Verification items for this drawing (mm, ordinates from the low corner). A direction names the side the tool comes from. Round coordinates to 2 decimals unless told otherwise and drop trailing zeros. Order: outer loops, then holes, each group sorted by start corner. A loop starts at its lowest first (then second) coordinate and runs counter-clockwise, first axis right, second up. Notation, with made-up numbers: (84, 85) -> (129, 85) arc R8 ccw to (129, 99) -> close; hole circle Ø5 at (-25, 27). An arc over 180 degrees is marked (long way). Answer in a Markdown table with one row per item. Add a question column.
1. Sectioned sample at B-B, the plane z = 12.7. Record the boundary of the cut face in (x, y) (1 decimal).
2. Access from +Z, -Z, +X, -X, +Y, -Y to the whole of each face (thin tool, end or side, straight path). Record for the marked faces 4 and 5.
3. Sectioned sample at C-C, the plane z = 19.75. Record the boundary of the cut face in (x, y) (1 decimal).
4. Sectioned sample at D-D, the plane x = 9.75. Record the boundary of the cut face in (y, z) (1 decimal).
5. Sectioned sample at A-A, the plane y = 12.7. Record the boundary of the cut face in (x, z) (1 decimal).
6. Draft check along X on the marked faces 1, 2 and 3. Enter one of: +X half, -X half, draft (parallel to the pull), parting line (faces both ways), or undercut.
7. Depth check by flat-ended pin: P1, Ø10, axis at x = 21, z = 14.5, coming from the +Y side (3 decimals); P2, Ø6, axis at y = 11.5, z = 14, coming from the +X side (3 decimals). Enter the tip coordinate at first touch or a pass-through.
8. Material ranges on L1, parallel to Y at x = 1.8, z = 12.7; L2, parallel to X at y = 2.4, z = 12.7 (1 decimal); L3, parallel to Y at x = 15.75, z = 2 (1 decimal), recorded low to high. Write a range as from..to.
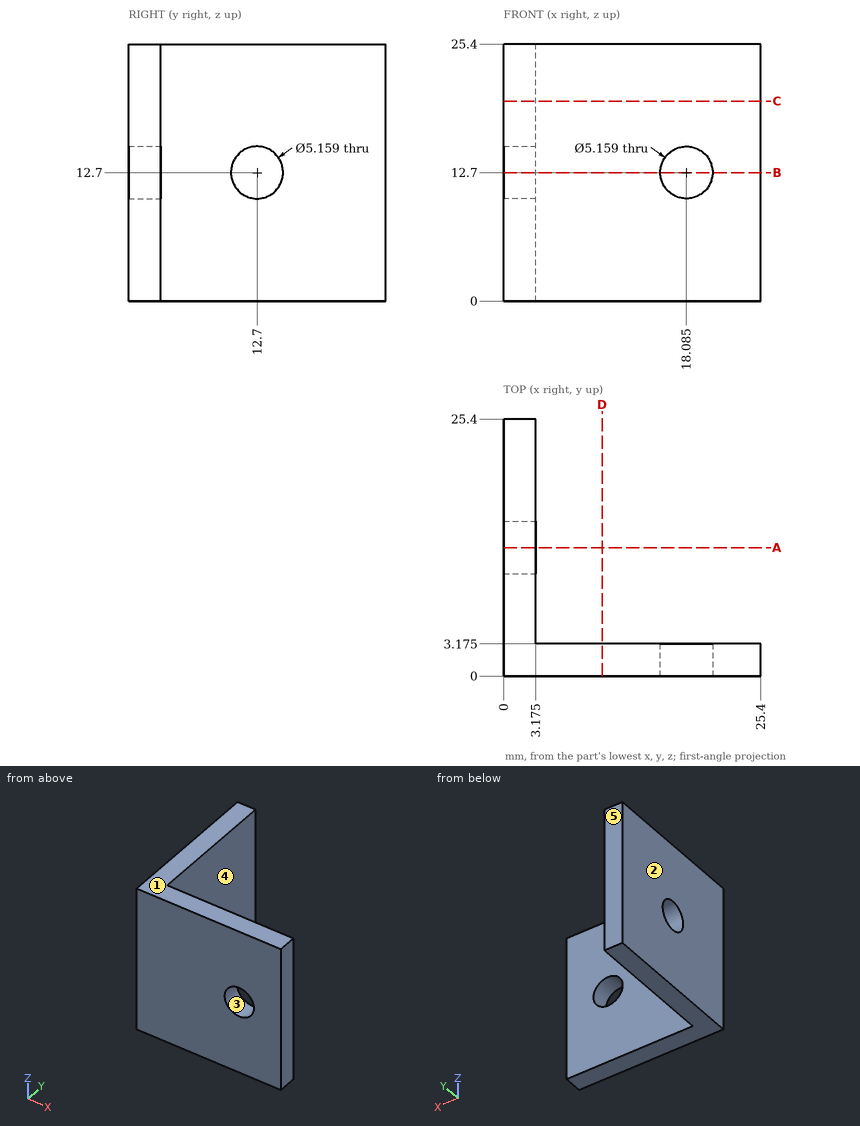
Answer key:
| question | item | result |
|---|---|---|
| 1 | outline | (0, 0) -> (15.5, 0) -> (15.5, 3.2) -> (3.2, 3.2) -> (3.2, 10.1) -> (0, 10.1) -> close; (0, 15.3) -> (3.2, 15.3) -> (3.2, 25.4) -> (0, 25.4) -> close; (20.7, 0) -> (25.4, 0) -> (25.4, 3.2) -> (20.7, 3.2) -> close |
| 2 | face 4 | +Z, -Z, +X, +Y |
| 2 | face 5 | +Z, -Z, +X, -X, +Y |
| 3 | outline | (0, 0) -> (25.4, 0) -> (25.4, 3.2) -> (3.2, 3.2) -> (3.2, 25.4) -> (0, 25.4) -> close |
| 4 | outline | (0, 0) -> (3.2, 0) -> (3.2, 25.4) -> (0, 25.4) -> close |
| 5 | outline | (0, 0) -> (3.2, 0) -> (3.2, 10.1) -> (0, 10.1) -> close; (0, 15.3) -> (3.2, 15.3) -> (3.2, 25.4) -> (0, 25.4) -> close |
| 6 | face 1 | draft |
| 6 | face 2 | -X half |
| 6 | face 3 | undercut |
| 7 | P1 | stops at y = 3.175 |
| 7 | P2 | stops at x = 3.175 |
| 8 | L1 | y = 0..10.12, 15.28..25.4 |
| 8 | L2 | x = 0..15.5, 20.7..25.4 |
| 8 | L3 | y = 0..3.2 |
